For this review, take the finished solid that the model builds, in its own axes (mm). Face numbers are marked on the shaded views. A direction names the side the tool comes from. Coordinates: 2 decimals unless noted, no trailing zeros. Loops run counter-clockwise (first coordinate to the right, second up) from the corner with the lowest first, then second, coordinate; pieces in that order, holes last. Notation, with made-up numbers: (27, -2) -> (39, -2) arc R9 cw to (39, 5) -> close; hole circle Ø2 at (11, 2). An arc over 180 degrees is marked (long way). Answer in a Markdown table with one row per item.
Autodesk Fusion 360 part; units mm, degrees
sketch "Sketch1" plane through (0, 0, 0) normal (0, 1, 0) x (1, 0, 0)
  line L0 (0, 0) -> (100, 0)
  line L1 (100, 0) -> (100, 60)
  line L2 (100, 60) -> (0, 60)
  line L3 (0, 60) -> (0, 0)
  dimension "d1" = 100
  dimension "d2" = 60
extrude "Extrude1" add sketch "Sketch1" along normal blind 3
sketch "Sketch2" plane through (0, 3, 0) normal (0, 1, 0) x (-1, 0, 0)
  line L0 (0, -60) -> (0, 0)
  line L1 (0, 0) -> (-100, 0)
  line L2 (-100, 0) -> (-100, -60)
  line L3 (-100, -60) -> (0, -60)
  line L4 (-5, -2) -> (-15, -2)
  line L5 (-15, -2) -> (-15, -4)
  line L6 (-15, -4) -> (-5, -4)
  line L7 (-5, -4) -> (-5, -2)
  line L8 (-25, -2) -> (-35, -2)
  line L9 (-35, -2) -> (-35, -4)
  line L10 (-35, -4) -> (-25, -4)
  line L11 (-25, -4) -> (-25, -2)
  line L12 (-45, -2) -> (-55, -2)
  line L13 (-55, -2) -> (-55, -4)
  line L14 (-55, -4) -> (-45, -4)
  line L15 (-45, -4) -> (-45, -2)
  line L16 (-65, -2) -> (-75, -2)
  line L17 (-75, -2) -> (-75, -4)
  line L18 (-75, -4) -> (-65, -4)
  line L19 (-65, -4) -> (-65, -2)
  line L20 (-5, -56) -> (-15, -56)
  line L21 (-15, -56) -> (-15, -58)
  line L22 (-15, -58) -> (-5, -58)
  line L23 (-5, -58) -> (-5, -56)
  line L24 (-25, -56) -> (-35, -56)
  line L25 (-35, -56) -> (-35, -58)
  line L26 (-35, -58) -> (-25, -58)
  line L27 (-25, -58) -> (-25, -56)
  line L28 (-45, -56) -> (-55, -56)
  line L29 (-55, -56) -> (-55, -58)
  line L30 (-55, -58) -> (-45, -58)
  line L31 (-45, -58) -> (-45, -56)
  line L32 (-65, -56) -> (-75, -56)
  line L33 (-75, -56) -> (-75, -58)
  line L34 (-75, -58) -> (-65, -58)
  line L35 (-65, -58) -> (-65, -56)
  line L36 (-4, -5) -> (-2, -5)
  line L37 (-2, -5) -> (-2, -15)
  line L38 (-2, -15) -> (-4, -15)
  line L39 (-4, -15) -> (-4, -5)
  line L40 (-98, -15) -> (-98, -5)
  line L41 (-98, -5) -> (-96, -5)
  line L42 (-96, -5) -> (-96, -15)
  line L43 (-96, -15) -> (-98, -15)
  line L44 (-4, -35) -> (-4, -25)
  line L45 (-4, -25) -> (-2, -25)
  line L46 (-2, -25) -> (-2, -35)
  line L47 (-2, -35) -> (-4, -35)
  line L48 (-98, -35) -> (-98, -25)
  line L49 (-98, -25) -> (-96, -25)
  line L50 (-96, -25) -> (-96, -35)
  line L51 (-96, -35) -> (-98, -35)
  line L52 (-85, -2) -> (-95, -2)
  line L53 (-95, -2) -> (-95, -4)
  line L54 (-95, -4) -> (-85, -4)
  line L55 (-85, -4) -> (-85, -2)
  line L56 (-85, -56) -> (-95, -56)
  line L57 (-95, -56) -> (-95, -58)
  line L58 (-95, -58) -> (-85, -58)
  line L59 (-85, -58) -> (-85, -56)
  line L60 (-4, -55) -> (-4, -45)
  line L61 (-4, -45) -> (-2, -45)
  line L62 (-2, -45) -> (-2, -55)
  line L63 (-2, -55) -> (-4, -55)
  line L64 (-98, -55) -> (-98, -45)
  line L65 (-98, -45) -> (-96, -45)
  line L66 (-96, -45) -> (-96, -55)
  line L67 (-96, -55) -> (-98, -55)
  dimension "d5" = 2
  dimension "d6" = 5
  dimension "d7" = 10
  dimension "d8" = 2
  dimension "d11" = -20
  dimension "d12" = -54
  dimension "d13" = 2
  dimension "d14" = 2
  dimension "d15" = 5
  dimension "d16" = 10
  dimension "d19" = -94
  dimension "d20" = -20
extrude "Extrude2" cut sketch "Sketch2" against normal blind 3 contours L4 L5 L6 L7 | L8 L9 L10 L11 | L12 L13 L14 L15 | L16 L17 L18 L19 | L20 L21 L22 L23 | L24 L25 L26 L27 | L28 L29 L30 L31 | L32 L33 L34 L35 | L36 L37 L38 L39 | L40 L41 L42 L43 | L44 L45 L46 L47 | L48 L49 L50 L51 | L52 L53 L54 L55 | L56 L57 L58 L59 | L60 L61 L62 L63 | L64 L65 L66 L67
sketch "Sketch3" plane through (0, 3, 0) normal (0, 1, 0) x (-1, 0, 0)
  line L0 (-4, -25) -> (-2, -25)
  line L1 (-2, -25) -> (-2, -35)
  line L2 (-2, -35) -> (-4, -35)
  line L3 (-4, -35) -> (-4, -25)
  line L4 (-75, -2) -> (-65, -2)
  line L5 (-65, -2) -> (-65, -4)
  line L6 (-65, -4) -> (-75, -4)
  line L7 (-75, -4) -> (-75, -2)
  line L8 (-55, -2) -> (-45, -2)
  line L9 (-45, -2) -> (-45, -4)
  line L10 (-45, -4) -> (-55, -4)
  line L11 (-55, -4) -> (-55, -2)
  line L12 (-2, -5) -> (-2, -15)
  line L13 (-2, -15) -> (-4, -15)
  line L14 (-4, -15) -> (-4, -5)
  line L15 (-4, -5) -> (-2, -5)
  line L16 (-15, -56) -> (-5, -56)
  line L17 (-5, -56) -> (-5, -58)
  line L18 (-5, -58) -> (-15, -58)
  line L19 (-15, -58) -> (-15, -56)
  line L20 (-55, -56) -> (-45, -56)
  line L21 (-45, -56) -> (-45, -58)
  line L22 (-45, -58) -> (-55, -58)
  line L23 (-55, -58) -> (-55, -56)
  line L24 (-75, -56) -> (-65, -56)
  line L25 (-65, -56) -> (-65, -58)
  line L26 (-65, -58) -> (-75, -58)
  line L27 (-75, -58) -> (-75, -56)
  line L28 (-15, -2) -> (-5, -2)
  line L29 (-5, -2) -> (-5, -4)
  line L30 (-5, -4) -> (-15, -4)
  line L31 (-15, -4) -> (-15, -2)
  line L32 (-35, -56) -> (-25, -56)
  line L33 (-25, -56) -> (-25, -58)
  line L34 (-25, -58) -> (-35, -58)
  line L35 (-35, -58) -> (-35, -56)
  line L36 (-98, -25) -> (-96, -25)
  line L37 (-96, -25) -> (-96, -35)
  line L38 (-96, -35) -> (-98, -35)
  line L39 (-98, -35) -> (-98, -25)
  line L40 (-35, -2) -> (-25, -2)
  line L41 (-25, -2) -> (-25, -4)
  line L42 (-25, -4) -> (-35, -4)
  line L43 (-35, -4) -> (-35, -2)
  line L44 (-98, -5) -> (-96, -5)
  line L45 (-96, -5) -> (-96, -15)
  line L46 (-96, -15) -> (-98, -15)
  line L47 (-98, -15) -> (-98, -5)
  line L48 (0, -60) -> (0, 0)
  line L49 (0, 0) -> (-100, 0)
  line L50 (-100, 0) -> (-100, -60)
  line L51 (-100, -60) -> (0, -60)
  circle A0 centre (-10, -10) radius 1.5
  circle A1 centre (-85.5, -10) radius 1.5
  line L52 (-95, -56) -> (-85, -56)
  line L53 (-85, -56) -> (-85, -58)
  line L54 (-85, -58) -> (-95, -58)
  line L55 (-95, -58) -> (-95, -56)
  line L56 (-95, -2) -> (-85, -2)
  line L57 (-85, -2) -> (-85, -4)
  line L58 (-85, -4) -> (-95, -4)
  line L59 (-95, -4) -> (-95, -2)
  circle A2 centre (-10, -40.5) radius 1.5
  circle A3 centre (-85.5, -40.5) radius 1.5
  line L60 (-4, -45) -> (-2, -45)
  line L61 (-2, -45) -> (-2, -55)
  line L62 (-2, -55) -> (-4, -55)
  line L63 (-4, -55) -> (-4, -45)
  line L64 (-98, -45) -> (-96, -45)
  line L65 (-96, -45) -> (-96, -55)
  line L66 (-96, -55) -> (-98, -55)
  line L67 (-98, -55) -> (-98, -45)
  dimension "d23" = 75.5
  dimension "d24" = 30.5
  dimension "d25" = 10
  dimension "d26" = 10
  dimension "d27" = 3
  dimension "d28" = 3
  dimension "d29" = 3
  dimension "d30" = 3
extrude "Extrude3" cut sketch "Sketch3" against normal blind 3 contours A0 | A1 | A2 | A3
sketch "Sketch4" plane through (0, 3, 0) normal (0, 1, 0) x (-1, 0, 0)
  circle A0 centre (-10, -40.5) radius 1.5
  circle A1 centre (-85.5, -40.5) radius 1.5
  circle A2 centre (-10, -10) radius 1.5
  circle A3 centre (-85.5, -10) radius 1.5
  line L0 (-95, -2) -> (-85, -2)
  line L1 (-85, -2) -> (-85, -4)
  line L2 (-85, -4) -> (-95, -4)
  line L3 (-95, -4) -> (-95, -2)
  line L4 (-4, -25) -> (-2, -25)
  line L5 (-2, -25) -> (-2, -35)
  line L6 (-2, -35) -> (-4, -35)
  line L7 (-4, -35) -> (-4, -25)
  line L8 (-75, -2) -> (-65, -2)
  line L9 (-65, -2) -> (-65, -4)
  line L10 (-65, -4) -> (-75, -4)
  line L11 (-75, -4) -> (-75, -2)
  line L12 (-55, -2) -> (-45, -2)
  line L13 (-45, -2) -> (-45, -4)
  line L14 (-45, -4) -> (-55, -4)
  line L15 (-55, -4) -> (-55, -2)
  line L16 (-2, -5) -> (-2, -15)
  line L17 (-2, -15) -> (-4, -15)
  line L18 (-4, -15) -> (-4, -5)
  line L19 (-4, -5) -> (-2, -5)
  line L20 (-15, -56) -> (-5, -56)
  line L21 (-5, -56) -> (-5, -58)
  line L22 (-5, -58) -> (-15, -58)
  line L23 (-15, -58) -> (-15, -56)
  line L24 (-55, -56) -> (-45, -56)
  line L25 (-45, -56) -> (-45, -58)
  line L26 (-45, -58) -> (-55, -58)
  line L27 (-55, -58) -> (-55, -56)
  line L28 (-4, -45) -> (-2, -45)
  line L29 (-2, -45) -> (-2, -55)
  line L30 (-2, -55) -> (-4, -55)
  line L31 (-4, -55) -> (-4, -45)
  line L32 (-95, -56) -> (-85, -56)
  line L33 (-85, -56) -> (-85, -58)
  line L34 (-85, -58) -> (-95, -58)
  line L35 (-95, -58) -> (-95, -56)
  line L36 (-75, -56) -> (-65, -56)
  line L37 (-65, -56) -> (-65, -58)
  line L38 (-65, -58) -> (-75, -58)
  line L39 (-75, -58) -> (-75, -56)
  line L40 (-15, -2) -> (-5, -2)
  line L41 (-5, -2) -> (-5, -4)
  line L42 (-5, -4) -> (-15, -4)
  line L43 (-15, -4) -> (-15, -2)
  line L44 (-35, -56) -> (-25, -56)
  line L45 (-25, -56) -> (-25, -58)
  line L46 (-25, -58) -> (-35, -58)
  line L47 (-35, -58) -> (-35, -56)
  line L48 (-98, -25) -> (-96, -25)
  line L49 (-96, -25) -> (-96, -35)
  line L50 (-96, -35) -> (-98, -35)
  line L51 (-98, -35) -> (-98, -25)
  line L52 (-35, -2) -> (-25, -2)
  line L53 (-25, -2) -> (-25, -4)
  line L54 (-25, -4) -> (-35, -4)
  line L55 (-35, -4) -> (-35, -2)
  line L56 (-98, -5) -> (-96, -5)
  line L57 (-96, -5) -> (-96, -15)
  line L58 (-96, -15) -> (-98, -15)
  line L59 (-98, -15) -> (-98, -5)
  line L60 (-98, -45) -> (-96, -45)
  line L61 (-96, -45) -> (-96, -55)
  line L62 (-96, -55) -> (-98, -55)
  line L63 (-98, -55) -> (-98, -45)
  line L64 (0, -60) -> (0, 0)
  line L65 (0, 0) -> (-100, 0)
  line L66 (-100, 0) -> (-100, -60)
  line L67 (-100, -60) -> (0, -60)
  circle A4 centre (-10, -10) radius 2.5
  circle A5 centre (-10, -40.5) radius 2.5
  circle A6 centre (-85.5, -40.5) radius 2.5
  circle A7 centre (-85.5, -10) radius 2.5
  dimension "d33" = 5
  dimension "d34" = 5
  dimension "d35" = 5
  dimension "d36" = 5
extrude "Extrude4" add sketch "Sketch4" along normal blind 3.5 contours A4 | A5 | A6 | A7
sketch "Sketch5" plane through (0, 3, 0) normal (0, 1, 0) x (-1, 0, 0)
  circle A0 centre (-85.5, -10) radius 2.5
  circle A1 centre (-10, -40.5) radius 2.5
  circle A2 centre (-85.5, -40.5) radius 2.5
  circle A3 centre (-10, -10) radius 2.5
  line L0 (-95, -2) -> (-85, -2)
  line L1 (-85, -2) -> (-85, -4)
  line L2 (-85, -4) -> (-95, -4)
  line L3 (-95, -4) -> (-95, -2)
  line L4 (-4, -25) -> (-2, -25)
  line L5 (-2, -25) -> (-2, -35)
  line L6 (-2, -35) -> (-4, -35)
  line L7 (-4, -35) -> (-4, -25)
  line L8 (-75, -2) -> (-65, -2)
  line L9 (-65, -2) -> (-65, -4)
  line L10 (-65, -4) -> (-75, -4)
  line L11 (-75, -4) -> (-75, -2)
  line L12 (-55, -2) -> (-45, -2)
  line L13 (-45, -2) -> (-45, -4)
  line L14 (-45, -4) -> (-55, -4)
  line L15 (-55, -4) -> (-55, -2)
  line L16 (-2, -5) -> (-2, -15)
  line L17 (-2, -15) -> (-4, -15)
  line L18 (-4, -15) -> (-4, -5)
  line L19 (-4, -5) -> (-2, -5)
  line L20 (-15, -56) -> (-5, -56)
  line L21 (-5, -56) -> (-5, -58)
  line L22 (-5, -58) -> (-15, -58)
  line L23 (-15, -58) -> (-15, -56)
  line L24 (-55, -56) -> (-45, -56)
  line L25 (-45, -56) -> (-45, -58)
  line L26 (-45, -58) -> (-55, -58)
  line L27 (-55, -58) -> (-55, -56)
  line L28 (-4, -45) -> (-2, -45)
  line L29 (-2, -45) -> (-2, -55)
  line L30 (-2, -55) -> (-4, -55)
  line L31 (-4, -55) -> (-4, -45)
  line L32 (-95, -56) -> (-85, -56)
  line L33 (-85, -56) -> (-85, -58)
  line L34 (-85, -58) -> (-95, -58)
  line L35 (-95, -58) -> (-95, -56)
  line L36 (-75, -56) -> (-65, -56)
  line L37 (-65, -56) -> (-65, -58)
  line L38 (-65, -58) -> (-75, -58)
  line L39 (-75, -58) -> (-75, -56)
  line L40 (-15, -2) -> (-5, -2)
  line L41 (-5, -2) -> (-5, -4)
  line L42 (-5, -4) -> (-15, -4)
  line L43 (-15, -4) -> (-15, -2)
  line L44 (-35, -56) -> (-25, -56)
  line L45 (-25, -56) -> (-25, -58)
  line L46 (-25, -58) -> (-35, -58)
  line L47 (-35, -58) -> (-35, -56)
  line L48 (-98, -25) -> (-96, -25)
  line L49 (-96, -25) -> (-96, -35)
  line L50 (-96, -35) -> (-98, -35)
  line L51 (-98, -35) -> (-98, -25)
  line L52 (-35, -2) -> (-25, -2)
  line L53 (-25, -2) -> (-25, -4)
  line L54 (-25, -4) -> (-35, -4)
  line L55 (-35, -4) -> (-35, -2)
  line L56 (-98, -5) -> (-96, -5)
  line L57 (-96, -5) -> (-96, -15)
  line L58 (-96, -15) -> (-98, -15)
  line L59 (-98, -15) -> (-98, -5)
  line L60 (-98, -45) -> (-96, -45)
  line L61 (-96, -45) -> (-96, -55)
  line L62 (-96, -55) -> (-98, -55)
  line L63 (-98, -55) -> (-98, -45)
  line L64 (0, -60) -> (0, 0)
  line L65 (0, 0) -> (-100, 0)
  line L66 (-100, 0) -> (-100, -60)
  line L67 (-100, -60) -> (0, -60)
  line L68 (-81.5, -6) -> (-14, -6)
  line L69 (-14, -6) -> (-14, -44.5)
  line L70 (-14, -44.5) -> (-81.5, -44.5)
  line L71 (-81.5, -44.5) -> (-81.5, -6)
  dimension "d39" = 4
  dimension "d40" = 6
  dimension "d42" = 15.5
  dimension "d43" = 4
extrude "Extrude5" cut sketch "Sketch5" against normal blind 3 contours L68 L69 L70 L71
fillet "Fillet1" radius 1.5 4 edges at (12.3308, 3, -9.096) (12.3308, 3, -39.596) (87.8308, 3, -39.596) (87.8308, 3, -9.096)
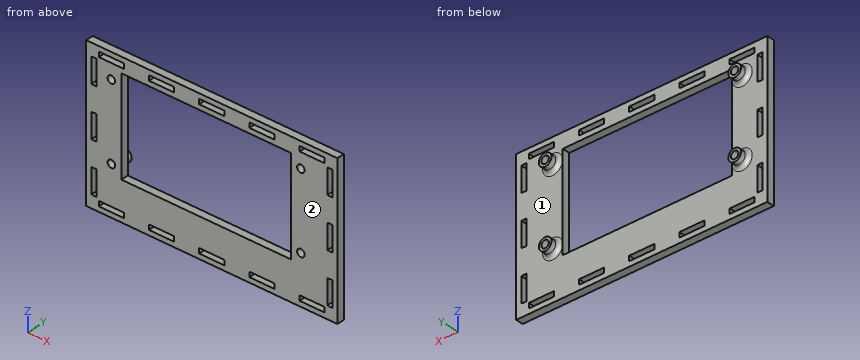
Item 1: For L1, parallel to Z at x = 7.5, y = 1.25; L2, parallel to X at y = 1.75, z = -12; L3, parallel to Z at x = 10, y = 1.5, list the stretches that pass through material, from the lowest coordinate up.
Worked answers:
| item | result |
|---|---|
| L1 | -60 to -58, -56 to -4, -2 to 0 |
| L2 | 0 to 2, 4 to 14, 81.5 to 96, 98 to 100 |
| L3 | -60 to -58, -56 to -42, -39 to -11.5, -8.5 to -4, -2 to 0 |
Item 2: For the marked faces 1 and 2, list the 3-axis set-ups (+Z, -Z, +X, -X, +Y, -Y) from which the entire face can be reached by the end or side of a thin tool; tool diameter is ignored.
Worked answers:
| item | result |
|---|---|
| face 1 | +Y |
| face 2 | +Z, -Z, +X, -X, -Y |
Item 3: Insertion check: pin 1 (1.5 mm diameter, centred on x = 62.5, z = -49, fed in from +Y). The pin has a flat end and moves straight along its axis. Give the tip position at first contact, or say it passes through.
Worked answers:
| item | result |
|---|---|
| pin 1 | y = 3 |
Item 4: Take a section at A-A, the plane y = 5.5. State the section outline as (x, z) points, and give its area (3 significant figures).
Worked answers:
| item | result |
|---|---|
| outline | circle Ø5 at (10, -40.5); circle Ø5 at (10, -10); circle Ø5 at (85.5, -40.5); circle Ø5 at (85.5, -10); hole circle Ø3 at (10, -40.5); hole circle Ø3 at (10, -10); hole circle Ø3 at (85.5, -40.5); hole circle Ø3 at (85.5, -10) |
| area | 50.3 mm² |
Item 5: Take a section at C-C, the plane z = -30. State the section outline as (x, y) points.
Worked answers:
| item | result |
|---|---|
| outline | (0, 0) -> (2, 0) -> (2, 3) -> (0, 3) -> close; (4, 0) -> (14, 0) -> (14, 3) -> (4, 3) -> close; (81.5, 0) -> (96, 0) -> (96, 3) -> (81.5, 3) -> close; (98, 0) -> (100, 0) -> (100, 3) -> (98, 3) -> close |
Item 6: Take a section at D-D, the plane x = 10. Count the separate pieces of the cut face and the enclosed holes in it, and give its area (3 significant figures).
Worked answers:
| item | result |
|---|---|
| separate pieces | 5 |
| enclosed holes | 0 |
| area | 166 mm² |
Item 7: Take a section at B-B, the plane x = 27. State the section outline as (y, z) points.
Worked answers:
| item | result |
|---|---|
| outline | (0, -60) -> (3, -60) -> (3, -58) -> (0, -58) -> close; (0, -56) -> (3, -56) -> (3, -44.5) -> (0, -44.5) -> close; (0, -6) -> (3, -6) -> (3, -4) -> (0, -4) -> close; (0, -2) -> (3, -2) -> (3, 0) -> (0, 0) -> close |
